For this review, take the finished solid that the model builds, in its own axes (mm). A direction names the side the tool comes from. Coordinates: 2 decimals unless noted, no trailing zeros. Loops run counter-clockwise (first coordinate to the right, second up) from the corner with the lowest first, then second, coordinate; pieces in that order, holes last. Notation, with made-up numbers: (54, 67.5) - (102, 67.5) arc R24 cw to (102, 96.5) - close; hole circle Ø1 at (-33.75, -19.75). An arc over 180 degrees is marked (long way). Answer as a JSON object with one key per item and string values. Group by question number.
Item 1: We need section B-B (z = 3.6). Give the boundary of the cut face in (x, y), then the cut area to 3 significant figures.
Item 2: Mouldability with a two-part tool opening along Y and no side actions: class faces 4 (the flat face through (-2, 0, 5)), 5 (the flat face through (0, 1, 3)), 6 (the flat face through (-4, -2.5, 2)) as released by +Y, released by -Y, zero draft, split by the parting line, or undercut.
Item 3: We need section A-A (y = 0.6). Give the boundary of the cut face in (x, z).
Item 4: We need section C-C (x = 0.5). Give the boundary of the cut face in (y, z).
Item 5: To check wall thickness, follow line 1 (X direction, y = -0.6, z = 2.1); line 2 (X direction, y = -1.3, z = 0.6). State the ranges of each line that lie inside material, in increasing order.
Item 6: Tool access review of faces 1 (the flat face through (6.75, 0, 2)), 2 (the flat face through (1, -1, 3)), 3 (the cylindrical face through (0.914, -1.74, 2.535)): name each direction out of +Z, -Z, +X, -X, +Y, -Y from which nothing blocks a thin tool from reaching the whole face with its end or side.
from build123d import *

# Parameters (mm, degrees)
F0_W     = 13.5
F0_H     = 5
F1_DEPTH = 5
F3_DEPTH = 25


with BuildPart() as f1:
    # F0 (on Top) → F1 (new body)
    with BuildSketch(Plane.XY):
        Rectangle(F0_W, F0_H)
    extrude(amount=F1_DEPTH)

    # F2 (on face) → F3 (cut)
    with BuildSketch(Plane.XY.offset(5)):
        Polygon((1.5, -1), (1.5, 1), (-1.5, 1), (-1.5, -1), (-1, -1), (-1, 0.5), (1, 0.5), (1, -1), align=None)
        Polygon((0.65, -1), (1, -1), (1, 0.5), (-1, 0.5), (-1, -1), (-0.65, -1), align=None)
        with BuildLine():
            ThreePointArc((1, -2.5), (0.91134, -1.729854), (0.65, -1))
            Line((0.65, -1), (-0.65, -1))
            ThreePointArc((-0.65, -1), (-0.91134, -1.729854), (-1, -2.5))
            Line((-1, -2.5), (1, -2.5))
        make_face()
    extrude(amount=-F3_DEPTH, mode=Mode.SUBTRACT)


solid = f1.part
Check sheet entries:
{
 "1": {"outline": "(-6.75, -2.5) - (-1, -2.5) arc R3.39 cw to (-0.65, -1) - (-1.5, -1) - (-1.5, 1) - (1.5, 1) - (1.5, -1) - (0.65, -1) arc R3.39 cw to (1, -2.5) - (6.75, -2.5) - (6.75, 2.5) - (-6.75, 2.5) - close", "area": "58.8 mm2"},
 "2": {"face 4": "zero draft", "face 5": "undercut", "face 6": "released by -Y"},
 "3": {"outline": "(-6.75, 0) - (-1.5, 0) - (-1.5, 5) - (-6.75, 5) - close; (1.5, 0) - (6.75, 0) - (6.75, 5) - (1.5, 5) - close"},
 "4": {"outline": "(1, 0) - (2.5, 0) - (2.5, 5) - (1, 5) - close"},
 "5": {"line 1": "x = -6.75 to -1.5, 1.5 to 6.75", "line 2": "x = -6.75 to -0.78, 0.78 to 6.75"},
 "6": {"face 1": "+Z, -Z, +X, +Y, -Y", "face 2": "+Z, -Z", "face 3": "+Z, -Z, -Y"}
}
